```python
from build123d import *

# Parameters (mm, degrees)
ESQUISSE1_W             = 28
ESQUISSE1_H             = 4
BOSS_EXTRU_1_DEPTH      = 3.5
ESQUISSE2_R             = 3
BOSS_EXTRU_2_DEPTH      = 4
ESQUISSE3_R             = 2
ENL_V_MAT_EXTRU_1_DEPTH = 4
ENL_V_MAT_EXTRU_2_DEPTH = 4
ENL_V_MAT_EXTRU_3_DEPTH = 4


with BuildPart() as part:
    # Esquisse1 → Boss.-Extru.1 (new body)
    with BuildSketch(Plane(origin=(0, 0, 0), x_dir=(1, 0, 0), z_dir=(0, 1, 0))):
        with Locations((14, 2)):
            Rectangle(ESQUISSE1_W, ESQUISSE1_H)
    extrude(amount=BOSS_EXTRU_1_DEPTH)

    # Esquisse2 → Boss.-Extru.2 (add)
    with BuildSketch(Plane(origin=(0, 3.5, 0), x_dir=(1, 0, 0), z_dir=(0, 1, 0))):
        with Locations(Location((3, 1.840675307, 0), (0, 0, 270))):
            Circle(ESQUISSE2_R)
        with Locations(Location((25, 1.840675307, 0), (0, 0, 270))):
            Circle(ESQUISSE2_R)
    extrude(amount=-BOSS_EXTRU_2_DEPTH)

    # Esquisse3 → Enlèv. mat.-Extru.1 (cut)
    with BuildSketch(Plane(origin=(0, 3.5, 0), x_dir=(1, 0, 0), z_dir=(0, 1, 0))):
        with Locations(Location((3, 1.840675307, 0), (0, 0, 270))):
            Circle(ESQUISSE3_R)
        with Locations(Location((25, 1.840675307, 0), (0, 0, 270))):
            Circle(ESQUISSE3_R)
    extrude(amount=-ENL_V_MAT_EXTRU_1_DEPTH, mode=Mode.SUBTRACT)

    # Esquisse4 → Enlèv. mat.-Extru.2 (cut)
    with BuildSketch(Plane(origin=(0, 3.5, 0), x_dir=(1, 0, 0), z_dir=(0, 1, 0))):
        with BuildLine():
            Line((0.917377406, 4), (-0.491965761, 5.461248673))
            Line((-0.491965761, 5.461248673), (-4.245883295, 1.840675307))
            Line((-4.245883295, 1.840675307), (-0.73023333, -1.804454542))
            Line((-0.73023333, -1.804454542), (0.631052045, 0))
            ThreePointArc((0.631052045, 0), (0.007656422, 2.054871271), (0.917377406, 4))
        make_face()
    extrude(amount=-ENL_V_MAT_EXTRU_2_DEPTH, mode=Mode.SUBTRACT)

    # Esquisse5 → Enlèv. mat.-Extru.3 (cut)
    with BuildSketch(Plane(origin=(0, 3.5, 0), x_dir=(1, 0, 0), z_dir=(0, 1, 0))):
        with BuildLine():
            Line((27.082622594, 4), (30.63271591, 7.550093316))
            Line((30.63271591, 7.550093316), (35.597188908, 2.585620319))
            Line((35.597188908, 2.585620319), (29.60753561, -3.40403298))
            Line((29.60753561, -3.40403298), (27.368947955, 0))
            ThreePointArc((27.368947955, 0), (27.992343578, 2.054871271), (27.082622594, 4))
        make_face()
    extrude(amount=-ENL_V_MAT_EXTRU_3_DEPTH, mode=Mode.SUBTRACT)


solid = part.part
```
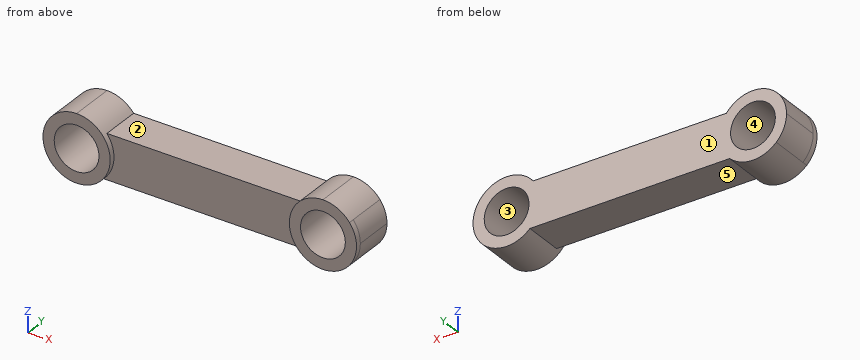
Can you work these out from the model? Positions are in its coordinate system, mm. Face numbers are marked on the shaded views. A direction names the side the tool comes from. Coordinates: 2 decimals unless noted, no trailing zeros. Write each loop counter-clockwise with the first axis right and the second up, starting at its lowest first coordinate (ties: lowest second). Pieces come first, ordered by that corner, then holes. Notation, with made-up numbers: M 49,65 L 80,65 A14 cw 80,80 Z; hole C 23,58 d9. An arc over 180 degrees is marked long. Write item = value, one per line. Start each with the question number.
Q1. I'm going to push flat-ended pins straight in: pin 1 (1 mm diameter, centred on x = 12, y = 1, fed in from -Z); pin 2 (1.8 mm diameter, centred on x = 14.5, y = 1.5, fed in from +Z); pin 3 (1.2 mm diameter, centred on x = 13.5, z = -3, fed in from -Y); pin 4 (2.5 mm diameter, centred on x = 25, z = -1.84, fed in from +Y). Where does each tip first touch, or does it pass through?
Q2. If we section it at B-B, the plane x = 25.5: Write out the boundary of the cut face in (y, z), then the cut area to 3 significant figures.
Q3. If we section it at D-D, the plane z = -4.4: Write out the boundary of the cut face in (x, y).
Q4. If we section it at A-A, the plane z = -3.2: Write out the boundary of the cut face in (x, y), then the cut area to 3 significant figures.
Q5. On a 3-axis mill with a long thin cutter (end or side, diameter ignored), from which of +Z, -Z, +X, -X, +Y, -Y can I reach the whole of each face in a straight line? I mean the marked faces 4 and 5. Say none if no direction works.
Q6. If I drill on L1, parallel to X at y = 1.6, z = -1.85; L2, parallel to X at y = 2.95, z = -2.75; L3, parallel to Z at x = 15, y = 3, over which ranges is the centre line in solid material (lowest first)? Write a range as [from, to].
Q7. Thinking about a two-plate mould opening in Z: for the marked faces 1, 2 and 3, which applies, released by +Z, released by -Z, zero draft, split by the parting line, or undercut?
Q8. If we section it at C-C, the plane y = 1.8: Write out the boundary of the cut face in (x, z).
Check sheet entries:
q1.pin_1 = -4
q1.pin_2 = 0
q1.pin_3 = 0
q1.pin_4 = through
q2.outline = M -0.5,-4.8 L 3.5,-4.8 L 3.5,-3.78 L -0.5,-3.78 Z; M -0.5,0.1 L 3.5,0.1 L 3.5,1.12 L -0.5,1.12 Z
q2.area = 8.17 mm²
q3.outline = M 1.43,-0.5 L 4.57,-0.5 L 4.57,3.5 L 1.43,3.5 Z; M 23.43,-0.5 L 26.57,-0.5 L 26.57,3.5 L 23.43,3.5 Z
q4.outline = M 0.33,-0.5 L 1.53,-0.5 L 1.53,3.5 L 0.33,3.5 Z; M 4.47,-0.5 L 5.67,-0.5 L 5.67,0 L 22.33,0 L 22.33,-0.5 L 23.53,-0.5 L 23.53,3.5 L 4.47,3.5 Z; M 26.47,-0.5 L 27.67,-0.5 L 27.67,3.5 L 26.47,3.5 Z
q4.area = 77.6 mm²
q5.face_4 = +Y, -Y
q5.face_5 = -Z, +Y, -Y
q6.L1 = [0, 1], [5, 23], [27, 28]
q6.L2 = [0.14, 1.22], [4.78, 23.22], [26.78, 27.86]
q6.L3 = [-4, 0]
q7.face_1 = zero draft
q7.face_2 = released by +Z
q7.face_3 = undercut
q8.outline = M 5.08,-4 L 22.92,-4 A3 ccw long 22.63,0 L 5.37,0 A3 ccw long Z; hole C 3,-1.84 d4; hole C 25,-1.84 d4
